Check sheet for the modelled part. Datum: model origin and axes. Units: mm. Round coordinates to 2 decimals unless told otherwise and drop trailing zeros. Write each loop counter-clockwise with the first axis right and the second up, starting at its lowest first coordinate (ties: lowest second). Pieces come first, ordered by that corner, then holes. Notation, with made-up numbers: (-26, -7.5) - (1, -7.5) arc R26 cw to (1, 6.5) - close; hole circle Ø7 at (-1.5, -34). An arc over 180 degrees is marked (long way). Answer as a JSON object with one key per item and string values. Group by question number.
Item 1: Release check for a two-part mould opening along X. For faces 1 (the flat face through (2, 10, -1.897)), 2 (the cylindrical face through (-13.29, -47.72, -0.94)) record: pulls with the +X half, pulls with the -X half, needs draft (parallel to the pull), parting line crosses it, or undercut.
Item 2: Thickness scan on line 1 (X direction, y = 66, z = -1); line 2 (Y direction, x = 13.5, z = -1.7); line 3 (Y direction, x = 58, z = -1.65). Record the ranges inside material, lowest first.
Item 3: Sectioned sample at A-A on x = 35. Record the boundary of the cut face in (y, z).
Item 4: Sectioned sample at B-B on x = -14.5. Record the boundary of the cut face in (y, z).
```python
from build123d import *

# Parameters (mm, degrees)
SKETCH1_W          = 100
SKETCH1_H          = 130
BASE_FLANGE1_DEPTH = 1.89738
SKETCH6_R          = 2.5
SKETCH6_R_2        = 2
CUT_EXTRUDE1_DEPTH = 2


# Sheet-metal steps are written as plain solids
with BuildPart() as part:
    # Sketch1 → Base-Flange1 (new body)
    with BuildSketch(Plane.XY):
        with Locations((14.222394098, 9.509380067)):
            Rectangle(SKETCH1_W, SKETCH1_H)
    extrude(amount=-BASE_FLANGE1_DEPTH)

    # Sketch6 → Cut-Extrude1 (cut)
    with BuildSketch(Plane.XY):
        with Locations((-34.133449647, 68.173545131)):
            Circle(SKETCH6_R)
        with Locations((55.866550353, 68.173545131)):
            Circle(SKETCH6_R)
        with Locations((35.363186693, -49.246493887)):
            Circle(SKETCH6_R)
        with Locations((-14.633449647, -49.826454869)):
            Circle(SKETCH6_R)
        with Locations((14.222394098, 9.509380067)):
            Circle(SKETCH6_R_2)
    extrude(amount=-CUT_EXTRUDE1_DEPTH, mode=Mode.SUBTRACT)


solid = part.part
```
Completed:
{
 "1": {"face 1": "needs draft", "face 2": "undercut"},
 "2": {"line 1": "-35.78 to -35.37, -32.9 to 54.63, 57.1 to 64.22", "line 2": "-55.49 to 7.64, 11.37 to 74.51", "line 3": "-55.49 to 66.87, 69.48 to 74.51"},
 "3": {"outline": "(-55.49, -1.9) - (-51.72, -1.9) - (-51.72, 0) - (-55.49, 0) - close; (-46.77, -1.9) - (74.51, -1.9) - (74.51, 0) - (-46.77, 0) - close"},
 "4": {"outline": "(-55.49, -1.9) - (-52.32, -1.9) - (-52.32, 0) - (-55.49, 0) - close; (-47.33, -1.9) - (74.51, -1.9) - (74.51, 0) - (-47.33, 0) - close"}
}
